CAD build for the part. Positions are in the model's coordinates, mm. A direction names the side the tool comes from. Give positions to 0.01 mm unless a question says otherwise; leave off trailing zeros. Order: outer loops, then holes, each group sorted by start corner. A loop starts at its lowest first (then second) coordinate and runs counter-clockwise, first axis right, second up. Notation, with made-up numbers: (43.5, 16) -> (59.5, 16) arc R28 ccw to (59.5, 50) -> close; hole circle Ø8 at (81, 1.25). An arc over 180 degrees is marked (long way). Use one line per item in the form item = value. Start each with the question number.
1) Cut at A-A, the plane z = -39. Give the cut face in (x, y).
2) Tool access for faces 5 (the face through (75, -25.4, -176)), 6 (the face through (12.7, -13, -64)): list every direction of +Z, -Z, +X, -X, +Y, -Y with a clear straight run to the whole face (end or side of a thin tool).
3) Probe line 1 (X direction, y = -22.25, z = -51); line 2 (X direction, y = -12.75, z = -105); line 3 (Z direction, x = 55, y = -12.75). List the from-to ranges inside material, lowest first.
4) Cut at C-C, the plane y = -22. State how many separate pieces and enclosed holes the cut face has, and give its area (3 significant figures).
5) Cut at B-B, the plane x = 158.75. Give the cut face in (y, z), and give its area (3 significant figures).
6) Drop flat-ended pins along their axis: P1, Ø8, axis at y = -3.5, z = -117, coming from the +X side; P2, Ø2, axis at y = -16.5, z = -191, coming from the +X side; P3, Ø2, axis at y = -12.5, z = -216, coming from the +X side. Give the stop position or say it passes through.
7) Mould opens along X. For faces 1 (the face through (153.244, -12.522, -278.796)), 2 (the face through (127, -13, -74)), 3 (the face through (5.73, -12.52, -5.43)), 4 (the face through (64, -13, -114.3)) say: pulls with the +X half, pulls with the -X half, needs draft (parallel to the pull), parting line crosses it, or undercut.
from build123d import *

# Parameters (mm, degrees)
F0_R     = 25.4
F1_DEPTH = 25.4


with BuildPart() as f1:
    # F0 (on Front) → F1 (new body)
    with BuildSketch(Plane.XZ):
        with BuildLine():
            Line((107.95, 0), (19.05, 0))
            ThreePointArc((19.05, 0), (5.579616, -5.579616), (0, -19.05))
            Line((0, -19.05), (0, -127))
            add(Edge.make_bspline(
                [(0, -127), (0, -200.66), (75.077975, -276.120124), (151.277975, -291.360124)],
                knots=[0, 0, 0, 0, 223.381459, 223.381459, 223.381459, 223.381459], degree=3))
            ThreePointArc((151.277975, -291.360124), (194.114391, -268.176383), (179.152879, -221.823417))
            ThreePointArc((179.152879, -221.823417), (140.898422, -181.109618), (127, -127))
            Line((127, -127), (127, -19.05))
            ThreePointArc((127, -19.05), (121.420384, -5.579616), (107.95, 0))
        make_face()
        with Locations((158.75, -254)):
            Circle(F0_R, mode=Mode.SUBTRACT)
        with BuildLine():
            Line((101.6, -114.3), (25.4, -114.3))
            ThreePointArc((25.4, -114.3), (16.419744, -110.580256), (12.7, -101.6))
            Line((12.7, -101.6), (12.7, -25.4))
            ThreePointArc((12.7, -25.4), (16.419744, -16.419744), (25.4, -12.7))
            Line((25.4, -12.7), (101.6, -12.7))
            ThreePointArc((101.6, -12.7), (110.580256, -16.419744), (114.3, -25.4))
            Line((114.3, -25.4), (114.3, -101.6))
            ThreePointArc((114.3, -101.6), (110.580256, -110.580256), (101.6, -114.3))
        make_face(mode=Mode.SUBTRACT)
    extrude(amount=F1_DEPTH)


solid = f1.part
Result:
q1.outline = (0, -25.4) -> (12.7, -25.4) -> (12.7, 0) -> (0, 0) -> close; (114.3, -25.4) -> (127, -25.4) -> (127, 0) -> (114.3, 0) -> close
q2.face_5 = +Z, -Z, +X, -X, -Y
q2.face_6 = +Y, -Y
q3.line_1 = 0 to 12.7, 114.3 to 127
q3.line_2 = 0 to 13.16, 113.84 to 127
q3.line_3 = -239.07 to -114.3, -12.7 to 0
q4.separate_pieces = 1
q4.enclosed_holes = 2
q4.area = 23,600 mm²
q5.outline = (-25.4, -292.1) -> (0, -292.1) -> (0, -279.4) -> (-25.4, -279.4) -> close; (-25.4, -228.6) -> (0, -228.6) -> (0, -205.24) -> (-25.4, -205.24) -> close
q5.area = 916 mm²
q6.P1 = 127
q6.P2 = 147.73
q6.P3 = 172.15
q7.face_1 = undercut
q7.face_2 = pulls with the +X half
q7.face_3 = pulls with the -X half
q7.face_4 = undercut
